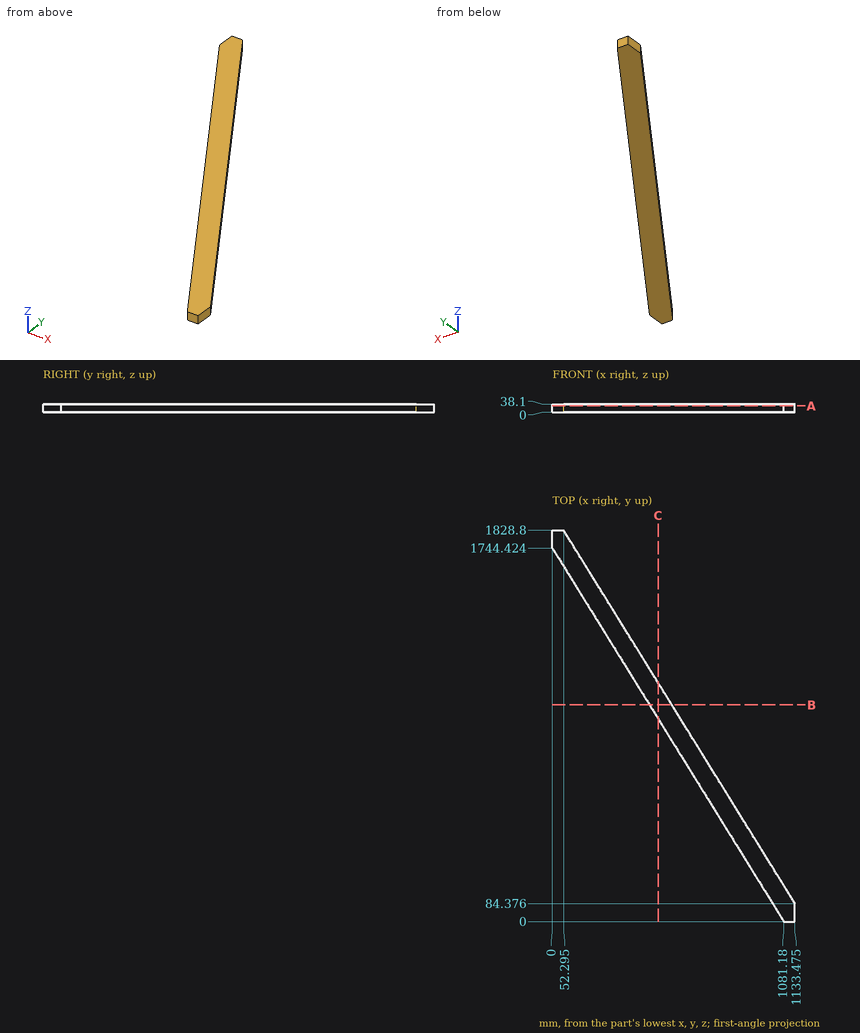
Can you work these out from the drawing? Everything is in mm from the part's minimum corner. Round coordinates to 2 decimals unless told otherwise and drop trailing zeros. Loops run counter-clockwise (first coordinate to the right, second up) from the corner with the lowest first, then second, coordinate; pieces in that order, holes last. Notation, with made-up numbers: M 65,33.25 L 107,33.25 A19 cw 107,54.25 Z; hole C 30.25,22.25 d5. An arc over 180 degrees is marked long. Answer in a Markdown table with one row per item.
1. If we section it at A-A, the plane z = 29: Please give me the cut outline in (x, y) (1 decimal).
Established:
| item | result |
|---|---|
| outline | M 0,1744.4 L 1081.2,0 L 1133.5,0 L 1133.5,84.4 L 52.3,1828.8 L 0,1828.8 Z |
2. If we section it at B-B, the plane y = 1012.5: Please give me the cut outline in (x, z).
Established:
| item | result |
|---|---|
| outline | M 453.64,0 L 558.23,0 L 558.23,38.1 L 453.64,38.1 Z |
3. Please list where these lines run through material, in increasing order: line 1 (Y direction, x = 789.5, z = 8); line 2 (X direction, y = 692.5, z = 31) (1 decimal); line 3 (X direction, y = 910, z = 32). Write a range as from..to.
Established:
| item | result |
|---|---|
| line 1 | 470.61..639.36 |
| line 2 | 652..756.6 |
| line 3 | 517.17..621.76 |
4. If we section it at C-C, the plane x = 493.5: Please give me the cut outline in (y, z), plus the area to 3 significant figures.
Established:
| item | result |
|---|---|
| outline | M 948.19,0 L 1116.94,0 L 1116.94,38.1 L 948.19,38.1 Z |
| area | 6,430 mm² |
5. I'm going to push flat-ended pins straight in: pin 1 Ø1.5 at (x, z) = (307.5, 30) entering from +Y; pin 2 Ø2 at (x, z) = (229, 20) entering from -Y; pin 3 Ø6 at (y, z) = (425, 10) entering from +X. Where does each tip first touch, or does it pass through?
Established:
| item | result |
|---|---|
| pin 1 | y = 1418.25 |
| pin 2 | y = 1373.33 |
| pin 3 | x = 924.22 |
